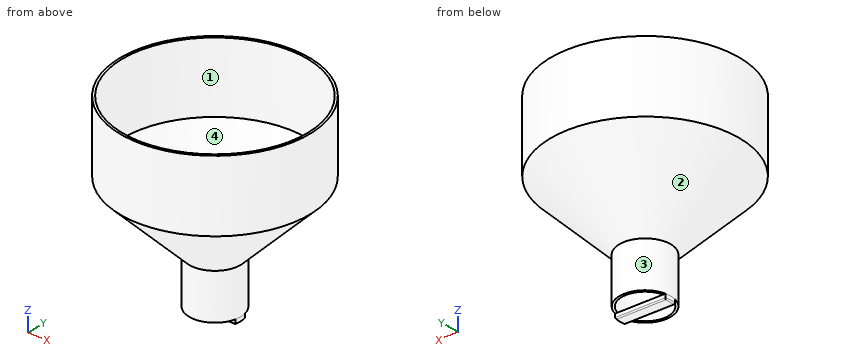
Autodesk Inventor part; units mm, degrees
ref_plane "YZ Plane" through (0, 0, 0) normal (1, 0, 0) x (0, 1, 0)
ref_plane "XZ Plane" through (0, 0, 0) normal (0, 1, 0) x (-1, 0, 0)
ref_plane "XY Plane" through (0, 0, 0) normal (0, 0, 1) x (1, 0, 0)
sketch "Sketch1" plane through (0, 0, 0) normal (1, 0, 0) x (0, 1, 0)
  line L0 (10, 0) -> (10, 20)
  line L1 (10, 20) -> (39.5, 49.5)
  line L2 (39.5, 49.5) -> (39.5, 79.5)
  line L3 (0, 79.5) -> (0, 0) construction
  line L4 (10, 20) -> (10, 79.5) construction
  line L5 (39.5, 79.5) -> (40.5, 79.5)
  line L6 (40.5, 79.5) -> (40.5, 49.0858)
  line L7 (40.5, 49.0858) -> (11, 19.5858)
  line L8 (11, 19.5858) -> (11, 0)
  line L9 (11, 0) -> (10, 0)
  dimension "Outlet_Height" = 20
  dimension "Funnel_Angle" = 45
  dimension "Inlet_Diameter" = 79
  dimension "Outlet_Diameter" = 20
  dimension "d23" = 1
  dimension "d24" = 1
  dimension "d25" = 1
  dimension "Inlet_Height" = 30
revolve "Revolution1" add sketch "Sketch1" angle 360 about axis through (0, 0, 79.5) along (0, 0, -1)
sketch "Sketch4" plane through (0, 0, 0) normal (0, 0, -1) x (-1, 0, 0)
  line L0 (0, 0) -> (-10.7121, 2.5) construction
  line L1 (0, 0) -> (-48.7838, 0) construction
  line L2 (0, 0) -> (-10.7121, -2.5) construction
  arc A0 (-10.7121, 2.5) -> (-10.7121, -2.5) centre (0, 0) ccw
  line L3 (0, 0) -> (0, 13.9156) construction
  arc A1 (10.7121, -2.5) -> (10.7121, 2.5) centre (0, 0) ccw
  line L4 (-10.7121, 2.5) -> (10.7121, 2.5)
  line L5 (10.7121, -2.5) -> (-10.7121, -2.5)
  circle A2 centre (0, 0) radius 11
  dimension "Bridge_Width" = 5
extrude "Extrusion1" add sketch "Sketch4" along normal blind 2 contours L4 A1 L5 A0
sketch "Sketch5" plane through (0, 0, -2) normal (0, 0, -1) x (-1, 0, 0)
  circle A0 centre (0, 0) radius 1.5
  dimension "Bridge_Hole" = 3
extrude "Extrusion2" [suppressed]
fillet "Fillet1" radius 0.5 4 edges at (11, 0, -2) (-11, 0, -2) (0, -2.5, -2) (0, 2.5, -2)
equation "\"d23\" = Wall_Thickness"
equation "\"d24\" = Wall_Thickness"
equation "\"d25\" = Wall_Thickness"
equation "\"Wall_Thickness\" = 1"
properties part number "Funnel"
The listing builds one solid part. Answer for the finished solid, in the listing's coordinates (mm). Face numbers are marked on the shaded views. A direction names the side the tool comes from. Coordinates: 2 decimals unless noted, no trailing zeros. Write each loop counter-clockwise with the first axis right and the second up, starting at its lowest first coordinate (ties: lowest second). Pieces come first, ordered by that corner, then holes. Notation, with made-up numbers: M 69.5,-16.5 L 101.5,-16.5 A26 ccw 101.5,5.5 Z; hole C 14,14.5 d1. An arc over 180 degrees is marked long. Use a Markdown table: item, result. Add a question column.
1. Section D-D (z = 71.5) is taken. Give the vertices of the cut face in (x, y).
2. Given P1, Ø1.5, axis at x = 1.5, y = -1, coming from the +Z side; P2, Ø2.5, axis at x = -3.5, y = 6, coming from the -Z side; P3, Ø4, axis at x = 4, y = -8.5, coming from the -Z side; P4, Ø8, axis at y = -8, z = 35, coming from the -X side, each flat-ended and moving along its own axis, determine where each tip first touches the part or whether it passes through.
3. Which of the six approach directions +Z, -Z, +X, -X, +Y, -Y give full straight-line access (tool end or side, diameter ignored) to the marked faces 3 and 4?
4. Section A-A (x = 0) is taken. Give the vertices of the cut face in (y, z).
5. Section C-C (z = 16.5) is taken. Give the vertices of the cut face in (x, y).
6. Section B-B (y = 0) is taken. Give the vertices of the cut face in (x, z), plus the area to 3 significant figures.
7. Straight lines are drawn through the part: line 1 along X through (y, z) = (0, 5); line 2 along X through (y, z) = (0, 71); line 3 along Y through (x, z) = (16.5, 75). For each, find the intervals that lie inside material, in ascending order. Write a range as [from, to].
8. For a pull along X with two mould halves and no side action, classify the marked faces 1 and 2 as +X half, -X half, draft (parallel to the pull), parting line (faces both ways), or undercut.
Data:
| question | item | result |
|---|---|---|
| 1 | outline | C 0,0 d81; hole C 0,0 d79 |
| 2 | P1 | stops at z = 0 |
| 2 | P2 | passes through |
| 2 | P3 | stops at z = 0 |
| 2 | P4 | stops at x = -29.47 |
| 3 | face 3 | -Z |
| 3 | face 4 | +Z |
| 4 | outline | M -40.5,49.09 L -11,19.59 L -11,0 L -10,0 L -10,20 L -39.5,49.5 L -39.5,79.5 L -40.5,79.5 Z; M -2.5,-1.5 A0.5 ccw -2,-2 L 2,-2 A0.5 ccw 2.5,-1.5 L 2.5,0 L -2.5,0 Z; M 10,0 L 11,0 L 11,19.59 L 40.5,49.09 L 40.5,79.5 L 39.5,79.5 L 39.5,49.5 L 10,20 Z |
| 5 | outline | C 0,0 d22; hole C 0,0 d20 |
| 6 | outline | M -40.5,49.09 L -11,19.59 L -11,-1.5 A0.5 ccw -10.5,-2 L 10.5,-2 A0.5 ccw 11,-1.5 L 11,19.59 L 40.5,49.09 L 40.5,79.5 L 39.5,79.5 L 39.5,49.5 L 10,20 L 10,0 L -10,0 L -10,20 L -39.5,49.5 L -39.5,79.5 L -40.5,79.5 Z |
| 6 | area | 227 mm2 |
| 7 | line 1 | x = [-11, -10], [10, 11] |
| 7 | line 2 | x = [-40.5, -39.5], [39.5, 40.5] |
| 7 | line 3 | y = [-36.99, -35.89], [35.89, 36.99] |
| 8 | face 1 | undercut |
| 8 | face 2 | parting line |
